Autodesk Fusion 360 part; units mm, degrees
sketch "Sketch1" plane through (0, 0, 0) normal (0, 1, 0) x (1, 0, 0)
  line L0 (0, 0) -> (15, 0)
  line L1 (15, 0) -> (15, -15)
  line L2 (15, -15) -> (0, -15)
  line L3 (0, -15) -> (0, 0)
  dimension "d1" = 15
  dimension "d2" = 15
extrude "Extrude1" add sketch "Sketch1" along normal blind 30
sketch "Sketch3" plane through (0, 0, 15) normal (0, 0, 1) x (-1, 0, 0)
  line L0 (0, 0) -> (-15, 0)
  line L1 (-15, 0) -> (-15, -30)
  line L2 (-15, -30) -> (0, -30)
  line L3 (0, -30) -> (0, 0)
  line L4 (0, 0) -> (-9.4343, 0)
  line L5 (-9.4343, 0) -> (-9.4343, -2.5)
  line L6 (-9.4343, -2.5) -> (0, -2.5)
  line L7 (0, -2.5) -> (0, 0)
  line L8 (0, 0) -> (-7.5, 0)
  line L9 (-7.5, 0) -> (-7.5, -11.3998)
  line L10 (-7.5, -11.3998) -> (-7.5, -2.5)
  line L11 (-7.5, -2.5) -> (-7.5, -7.5)
  circle A0 centre (-7.5, -7.5) radius 2.5
  dimension "d13" = 2.5
  dimension "d14" = 5
  dimension "d15" = 5
extrude "Extrude3" cut sketch "Sketch3" against normal blind 34 contours L9 L10 L11 A0 | L9 L10 L11 A0
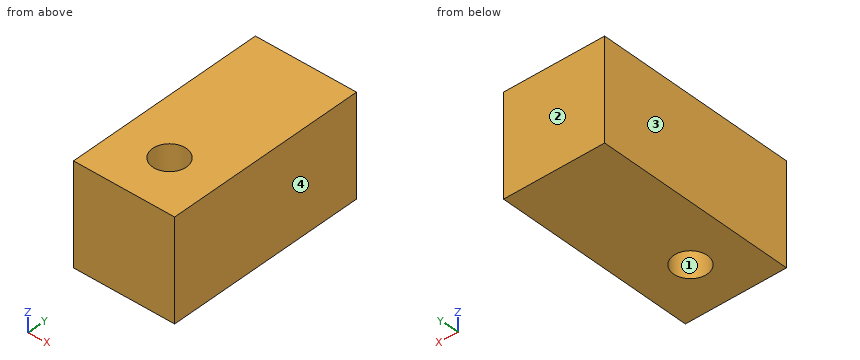
Geometry check sheet. Reference: the model listing, model coordinates, mm. Face numbers are marked on the shaded views. Give positions to 0.01 mm unless a question says otherwise; leave off trailing zeros. Loops run counter-clockwise (first coordinate to the right, second up) from the corner with the lowest first, then second, coordinate; pieces in that order, holes last. Notation, with made-up numbers: M 73.5,-37.75 L 80.5,-37.75 A13 cw 80.5,-22.75 Z; hole C -24,-20 d11. An arc over 180 degrees is marked long. Answer as a JSON object with one key per item and string values. Group by question number.
Item 1: Sectioned sample at C-C on z = 13.5. Record the boundary of the cut face in (x, y).
Item 2: Material ranges on L1, parallel to X at y = 7.5, z = 12; L2, parallel to Y at x = 7.5, z = 7.25; L3, parallel to Y at x = 8.5, z = 7.25, recorded low to high.
Item 3: Sectioned sample at B-B on y = 7.5. Record the boundary of the cut face in (x, z).
Item 4: Mould release check, pull along X, two halves, no side actions. Record for the marked faces 1, 2, 3 and 4: pulls with the +X half, pulls with the -X half, needs draft (parallel to the pull), parting line crosses it, or undercut.
Item 5: Sectioned sample at A-A on x = 7.5. Record the boundary of the cut face in (y, z), plus the area to 3 significant figures.
Findings below:
{
 "1": {"outline": "M 0,0 L 15,0 L 15,30 L 0,30 Z; hole C 7.5,7.5 d5"},
 "2": {"L1": "0 to 5, 10 to 15", "L2": "0 to 5, 10 to 30", "L3": "0 to 5.21, 9.79 to 30"},
 "3": {"outline": "M 0,0 L 5,0 L 5,15 L 0,15 Z; M 10,0 L 15,0 L 15,15 L 10,15 Z"},
 "4": {"face 1": "undercut", "face 2": "needs draft", "face 3": "pulls with the -X half", "face 4": "pulls with the +X half"},
 "5": {"outline": "M 0,0 L 5,0 L 5,15 L 0,15 Z; M 10,0 L 30,0 L 30,15 L 10,15 Z", "area": "375 mm2"}
}
